from build123d import *

# Parameters (mm, degrees)
F0_W        = 25.4
F0_H        = 50.8
F1_DEPTH    = 25.4
F3_DEPTH    = 50.8
F5_D        = 4.1
F6_F1_R     = 1.27
F6_F2_R     = 1.27
F7_T1_DEPTH = 23.8998895326


# Not quite as in the source:
# - a fillet or chamfer that OpenCascade refuses, or shapes differently, is made with other operations: its cross-section is extruded or revolved along the edge and cut away or added


with BuildPart() as f1:
    # F0 (on Top) → F1 (new body)
    with BuildSketch(Plane.XY):
        with Locations((12.7, -25.4)):
            Rectangle(F0_W, F0_H)
    extrude(amount=F1_DEPTH)

    # F2 (on face) → F3 (cut)
    with BuildSketch(Plane.XZ.offset(50.8)):
        with BuildLine():
            ThreePointArc((0, 25.4), (12.7, 12.7), (25.4, 25.4))
            Line((25.4, 25.4), (0, 25.4))
        make_face()
    extrude(amount=-F3_DEPTH, mode=Mode.SUBTRACT)

    # F5 (through all)
    with Locations(Plane(origin=(0, 0, 0), x_dir=(1, 0, 0), z_dir=(0, 0, -1))):
        with Locations((12.7, 25.4)):
            Hole(F5_D / 2)

    # F6: fillet of radius 1.27 on 2 edges, made by hand

    # F6_f1
    f6_f1_edges = [f1.edges().sort_by_distance(p)[0] for p in [
        (0, -25.4, 25.4),
    ]]
    fillet(f6_f1_edges, radius=F6_F1_R)

    # F6_f2
    f6_f2_edges = [f1.edges().sort_by_distance(p)[0] for p in [
        (25.4, -25.4, 25.4),
    ]]
    fillet(f6_f2_edges, radius=F6_F2_R)

    # F7: chamfer of 1.27 on 4 edges, made by hand

    # F7_s2 → F7_t1 (cut)
    with BuildSketch(Plane.XY.offset(-3.2660373947)):
        Polygon((25.4, -49.53), (24.13, -50.8), (25.4, -50.8), align=None)
        Polygon((0, -49.53), (1.27, -50.8), (0, -50.8), align=None)
        Polygon((24.13, 0), (25.4, -1.27), (25.4, 0), align=None)
        Polygon((1.27, 0), (0, -1.27), (0, 0), align=None)
    extrude(amount=F7_T1_DEPTH, mode=Mode.SUBTRACT)


solid = f1.part
The listing builds one solid part. Answer for the finished solid, in the listing's coordinates (mm). Give positions to 0.01 mm unless a question says otherwise; leave off trailing zeros. Write each loop counter-clockwise with the first axis right and the second up, starting at its lowest first coordinate (ties: lowest second). Pieces come first, ordered by that corner, then holes. Notation, with made-up numbers: (49, 45.5) -> (75, 45.5) arc R34 cw to (75, 79.5) -> close; hole circle Ø7 at (13, -1). An arc over 180 degrees is marked (long way). One line per question, with ' | ' between items. Start each with the question number.
1. For a pull along Y with two mould halves and no side action, classify faces 1 (the flat face through (0.64, -0.63, 9.19)), 2 (the flat face through (0, -26, 9)), 3 (the cylindrical face through (10.81, -24.61, 6.53)) as pulls with the +Y half, pulls with the -Y half, needs draft (parallel to the pull), parting line crosses it, or undercut.
2. Section B-B (y = -25.4) is taken. Determine the outline of the cut face in (x, z), plus the area to 3 significant figures.
3. Section C-C (z = 14.25) is taken. Determine the outline of the cut face in (x, y), plus the area to 3 significant figures.
4. Find the intervals of material crossed by probe 1 along Y at (x, z) = (12.7, 9.5); probe 2 along X at (y, z) = (-25.4, 8.25); probe 3 along X at (y, z) = (-5.5, 14.25), in increasing order.
5. Section A-A (x = 12.7) is taken. Determine the outline of the cut face in (y, z).
6. Given pin 1 Ø5.5 at (x, y) = (12.7, -25.4) entering from +Z; pin 2 Ø5 at (x, y) = (10, -18.5) entering from +Z, each flat-ended and moving along its own axis, determine where each tip first touches the part or whether it passes through.
7. Section D-D (y = -42.5) is taken. Determine the outline of the cut face in (x, z), plus the area to 3 significant figures.
Response values:
1) face 1: pulls with the +Y half | face 2: needs draft | face 3: undercut
2) outline: (0, 0) -> (10.65, 0) -> (10.65, 12.87) arc R12.7 cw to (2.31, 18.1) arc R1.27 ccw to (0, 17.37) -> close; (14.75, 0) -> (25.4, 0) -> (25.4, 17.37) arc R1.27 ccw to (23.09, 18.1) arc R12.7 cw to (14.75, 12.87) -> close | area: 330 mm2
3) outline: (0, -49.53) -> (1.27, -50.8) -> (6.62, -50.8) -> (6.62, 0) -> (1.27, 0) -> (0, -1.27) -> close; (18.78, -50.8) -> (24.13, -50.8) -> (25.4, -49.53) -> (25.4, -1.27) -> (24.13, 0) -> (18.78, 0) -> close | area: 669 mm2
4) probe 1: -50.8 to -27.45, -23.35 to 0 | probe 2: 0 to 10.65, 14.75 to 25.4 | probe 3: 0 to 6.62, 18.78 to 25.4
5) outline: (-50.8, 0) -> (-27.45, 0) -> (-27.45, 12.7) -> (-50.8, 12.7) -> close; (-23.35, 0) -> (0, 0) -> (0, 12.7) -> (-23.35, 12.7) -> close
6) pin 1: z = 13 | pin 2: z = 13.81
7) outline: (0, 0) -> (25.4, 0) -> (25.4, 17.37) arc R1.27 ccw to (23.09, 18.1) arc R12.7 cw to (2.31, 18.1) arc R1.27 ccw to (0, 17.37) -> close | area: 382 mm2
